Autodesk Inventor part; units mm, degrees
ref_plane "YZ Plane" through (0, 0, 0) normal (1, 0, 0) x (0, 1, 0)
ref_plane "XZ Plane" through (0, 0, 0) normal (0, 1, 0) x (-1, 0, 0)
ref_plane "XY Plane" through (0, 0, 0) normal (0, 0, 1) x (1, 0, 0)
sketch "Sketch1" plane through (0, 0, 0) normal (0, 0, 1) x (1, 0, 0)
  line L0 (-21, 33) -> (21, 33)
  line L1 (21, 33) -> (21, -33)
  line L2 (21, -33) -> (-21, -33)
  line L3 (-21, -33) -> (-21, 33)
  point P0 (0, 0)
  point P1 (0, 33)
  point P2 (-21, 0)
  dimension "d0" = 42
  dimension "d1" = 66
extrude "Extrusion1" add sketch "Sketch1" along normal blind 8
sketch "Sketch4" plane through (0, 0, 8) normal (0, 0, 1) x (1, 0, 0)
  line L0 (-21, -33) -> (21, -33)
  line L1 (21, 33) -> (-21, 33)
  line L2 (21, -33) -> (21, 33)
  point P0 (0, 0)
  point P1 (13, -29)
  point P2 (13, 29)
  dimension "d19" = 4
  dimension "d20" = 4
  dimension "d21" = 8
hole "Hole1" at (13, -29, 8) at (13, 29, 8) direction (0, 0, -1) diameter 4 end through all
properties part number "0005-10-016"
Verification items for the finished model (mm, model axes). Coordinates: 2 decimals unless noted, no trailing zeros. Order: outer loops, then holes, each group sorted by start corner. A loop starts at its lowest first (then second) coordinate and runs counter-clockwise, first axis right, second up. Notation, with made-up numbers: (36, 33) -> (53, 33) arc R9 cw to (53, 42) -> close; hole circle Ø11 at (-25, 48). An arc over 180 degrees is marked (long way). Put each result on its own line as item: value. Start each with the question number.
1. Mould release check, pull along Y, two halves, no side actions. Record for faces 1 (the flat face through (0, 33, 4)), 2 (the cylindrical face through (12.399, -30.908, 3.944)), 3 (the flat face through (21, 0, 4)): released by +Y, released by -Y, zero draft, split by the parting line, or undercut.
2. Cross-section at B-B, the plane y = 29. Record the boundary of the cut face in (x, z).
3. Cross-section at A-A, the plane x = 13. Record the boundary of the cut face in (y, z).
4. Material ranges on L1, parallel to Y at x = 13, z = 7.25; L2, parallel to X at y = 29, z = 2; L3, parallel to Y at x = 13.5, z = 6.25, recorded low to high. Write a range as [from, to].
Computed:
1. face 1: released by +Y
1. face 2: undercut
1. face 3: zero draft
2. outline: (-21, 0) -> (11, 0) -> (11, 8) -> (-21, 8) -> close; (15, 0) -> (21, 0) -> (21, 8) -> (15, 8) -> close
3. outline: (-33, 0) -> (-31, 0) -> (-31, 8) -> (-33, 8) -> close; (-27, 0) -> (27, 0) -> (27, 8) -> (-27, 8) -> close; (31, 0) -> (33, 0) -> (33, 8) -> (31, 8) -> close
4. L1: [-33, -31], [-27, 27], [31, 33]
4. L2: [-21, 11], [15, 21]
4. L3: [-33, -30.94], [-27.06, 27.06], [30.94, 33]
